For this review, take the finished solid that the model builds, in its own axes (mm). A direction names the side the tool comes from. Give positions to 0.01 mm unless a question says otherwise; leave off trailing zeros. Write each loop counter-clockwise with the first axis right and the second up, starting at its lowest first coordinate (ties: lowest second). Pieces come first, ordered by that corner, then holes.
1) Draft analysis for pull direction Z (two halves, no side actions). For faces 4 (the face through (7.509, 63.95, -23.846)), 5 (the face through (-19.04, 0, -10.33)), 6 (the face through (17, 140, 17)), 7 (the face through (-19, 45, -7)), state which applies: pulls with the +Z half, pulls with the -Z half, needs draft (parallel to the pull), parting line crosses it, or undercut.
2) Machinability: for faces 1 (the face through (-15.88, 20.71, 17.32)), 2 (the face through (-15.88, 91.84, 17.32)), 3 (the face through (-17, -10, -17)), which of the approach directions +Z, -Z, +X, -X, +Y, -Y give a long, thin tool a straight path to every point of the face, cutting with its end or side? Answer none if there is none.
3) We need section C-C on y = 47. Give the boundary of the cut face in (x, z).
4) We need section B-B on z = 0. Give the boundary of the cut face in (x, y).
5) For P1, Ø6, axis at y = 105, z = 9.5, coming from the -X side; P2, Ø12, axis at x = -10.5, y = 124, coming from the -Z side; P3, Ø8, axis at x = -5, z = -17.5, coming from the +Y side; P4, Ø15, axis at x = -4, z = 11.5, coming from the -Y side, all flat-tipped, find the tip position at first contact; note any pin that passes through.
6) We need section A-A on x = 0. Give the boundary of the cut face in (y, z), and give its area (3 significant figures).
7) Wall thickness on line 1 along X through (y, z) = (43.75, 0); line 2 along X through (y, z) = (29, 0); line 3 along Y through (x, z) = (-21, -11): over which ranges is each line inside the solid? List them lowest first.
from build123d import *

# Parameters (mm, degrees)
ESQUISSE1_R        = 25
ESQUISSE1_R_2      = 23.5
BOSS_EXTRU_1_DEPTH = 42
ESQUISSE4_R        = 25
ESQUISSE4_R_2      = 20
BOSS_EXTRU_4_DEPTH = 3
ESQUISSE5_R        = 25
ESQUISSE5_R_2      = 23.5
BOSS_EXTRU_5_DEPTH = 95
BOSS_EXTRU_6_START = 10
ESQUISSE7_R        = 25
ESQUISSE7_R_2      = 21.5
BOSS_EXTRU_6_DEPTH = 10
BOSS_EXTRU_7_START = 10
ESQUISSE8_R        = 23.4
ESQUISSE8_R_2      = 21.5
BOSS_EXTRU_7_DEPTH = 10


with BuildPart() as part:
    # Esquisse1 → Boss.-Extru.1 (new body)
    with BuildSketch(Plane(origin=(0, 0, 0), x_dir=(1, 0, 0), z_dir=(0, 1, 0))):
        with Locations(Location((0, 0, 0), (0, 0, 90))):
            Circle(ESQUISSE1_R)
        with Locations(Location((0, 0, 0), (0, 0, 90))):
            Circle(ESQUISSE1_R_2, mode=Mode.SUBTRACT)
    extrude(amount=BOSS_EXTRU_1_DEPTH)

    # Esquisse4 → Boss.-Extru.4 (add)
    with BuildSketch(Plane(origin=(0, 42, 0), x_dir=(1, 0, 0), z_dir=(0, 1, 0))):
        with Locations(Location((0, 0, 0), (0, 0, 90))):
            Circle(ESQUISSE4_R)
        with Locations(Location((0, 0, 0), (0, 0, 270))):
            Circle(ESQUISSE4_R_2, mode=Mode.SUBTRACT)
    extrude(amount=BOSS_EXTRU_4_DEPTH)

    # Esquisse5 → Boss.-Extru.5 (add)
    with BuildSketch(Plane(origin=(0, 45, 0), x_dir=(1, 0, 0), z_dir=(0, 1, 0))):
        with Locations(Location((0, 0, 0), (0, 0, 90))):
            Circle(ESQUISSE5_R)
        with Locations(Location((0, 0, 0), (0, 0, 90))):
            Circle(ESQUISSE5_R_2, mode=Mode.SUBTRACT)
    extrude(amount=BOSS_EXTRU_5_DEPTH)

    # Esquisse7 → Boss.-Extru.6 (add)
    with BuildSketch(Plane.XZ.offset(BOSS_EXTRU_6_START)):
        with Locations(Location((0, 0, 0), (0, 0, 270))):
            Circle(ESQUISSE7_R)
        with Locations(Location((0, 0, 0), (0, 0, 270))):
            Circle(ESQUISSE7_R_2, mode=Mode.SUBTRACT)
    extrude(amount=-BOSS_EXTRU_6_DEPTH)

    # Esquisse8 → Boss.-Extru.7 (add)
    with BuildSketch(Plane.XZ.offset(10).offset(BOSS_EXTRU_7_START)):
        with Locations(Location((0, 0, 0), (0, 0, 270))):
            Circle(ESQUISSE8_R)
        with Locations(Location((0, 0, 0), (0, 0, 270))):
            Circle(ESQUISSE8_R_2, mode=Mode.SUBTRACT)
    extrude(amount=-BOSS_EXTRU_7_DEPTH)


solid = part.part
Results list:
1. face 4: parting line crosses it
1. face 5: undercut
1. face 6: needs draft
1. face 7: undercut
2. face 1: none
2. face 2: +Y
2. face 3: -Y
3. outline: circle Ø50 at (0, 0); hole circle Ø47 at (0, 0)
4. outline: (-25, -10) - (-23.4, -10) - (-23.4, -20) - (-21.5, -20) - (-21.5, 0) - (-23.5, 0) - (-23.5, 42) - (-20, 42) - (-20, 45) - (-23.5, 45) - (-23.5, 140) - (-25, 140) - close; (20, 42) - (23.5, 42) - (23.5, 0) - (21.5, 0) - (21.5, -20) - (23.4, -20) - (23.4, -10) - (25, -10) - (25, 140) - (23.5, 140) - (23.5, 45) - (20, 45) - close
5. P1: stops at x = -24.14
5. P2: stops at z = -24.59
5. P3: stops at y = 45
5. P4: passes through
6. outline: (-20, -23.4) - (-10, -23.4) - (-10, -25) - (140, -25) - (140, -23.5) - (45, -23.5) - (45, -20) - (42, -20) - (42, -23.5) - (0, -23.5) - (0, -21.5) - (-20, -21.5) - close; (-20, 21.5) - (0, 21.5) - (0, 23.5) - (42, 23.5) - (42, 20) - (45, 20) - (45, 23.5) - (140, 23.5) - (140, 25) - (-10, 25) - (-10, 23.4) - (-20, 23.4) - close
6. area: 549 mm2
7. line 1: x = -25 to -20, 20 to 25
7. line 2: x = -25 to -23.5, 23.5 to 25
7. line 3: y = -10 to 140
